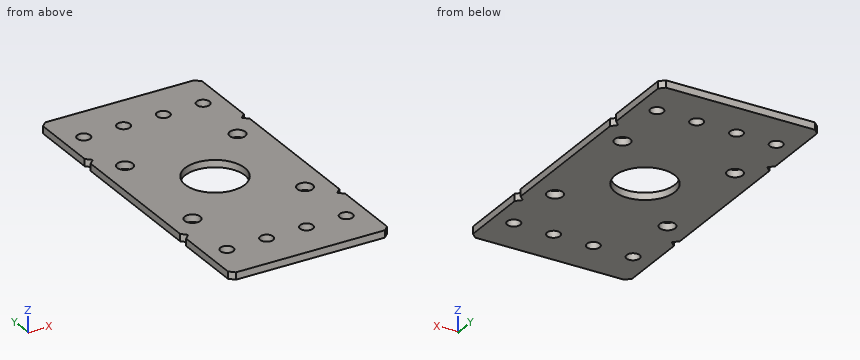
from build123d import *

# Parameters (mm, degrees)
SKETCH1_R           = 2.4892
SKETCH1_R_2         = 2.0701
SKETCH1_R_3         = 9.525
BOSS_EXTRUDE1_DEPTH = 2.286


with BuildPart() as part:
    # Sketch1 → Boss-Extrude1 (new body)
    with BuildSketch(Plane.XY.offset(2.286)):
        Polygon((25.4, -26.9875), (23.8125, -25.4), (25.4, -23.8125), (25.4, 23.8125), (23.8125, 25.4), (25.4, 26.9875), (25.4, 49.2125), (23.8125, 50.8), (-23.8125, 50.8), (-25.4, 49.2125), (-25.4, 26.9875), (-23.8125, 25.4), (-25.4, 23.8125), (-25.4, -23.8125), (-23.8125, -25.4), (-25.4, -26.9875), (-25.4, -49.2125), (-23.8125, -50.8), (23.8125, -50.8), (25.4, -49.2125), align=None)
        with Locations((-17.960512242, -17.960512242)):
            Circle(SKETCH1_R, mode=Mode.SUBTRACT)
        with Locations((-19.05, -38.1)):
            Circle(SKETCH1_R_2, mode=Mode.SUBTRACT)
        with Locations((-6.35, -38.1)):
            Circle(SKETCH1_R_2, mode=Mode.SUBTRACT)
        with Locations((19.05, -38.1)):
            Circle(SKETCH1_R_2, mode=Mode.SUBTRACT)
        Circle(SKETCH1_R_3, mode=Mode.SUBTRACT)
        with Locations((6.35, 38.1)):
            Circle(SKETCH1_R_2, mode=Mode.SUBTRACT)
        with Locations((-19.05, 38.1)):
            Circle(SKETCH1_R_2, mode=Mode.SUBTRACT)
        with Locations((-6.35, 38.1)):
            Circle(SKETCH1_R_2, mode=Mode.SUBTRACT)
        with Locations((19.05, 38.1)):
            Circle(SKETCH1_R_2, mode=Mode.SUBTRACT)
        with Locations((-17.960512242, 17.960512242)):
            Circle(SKETCH1_R, mode=Mode.SUBTRACT)
        with Locations((6.35, -38.1)):
            Circle(SKETCH1_R_2, mode=Mode.SUBTRACT)
        with Locations((17.960512242, -17.960512242)):
            Circle(SKETCH1_R, mode=Mode.SUBTRACT)
        with Locations((17.960512242, 17.960512242)):
            Circle(SKETCH1_R, mode=Mode.SUBTRACT)
    extrude(amount=-BOSS_EXTRUDE1_DEPTH)


solid = part.part
Geometry: final body of the model. Coordinates: model frame, mm. Give positions to 0.01 mm unless a question says otherwise; leave off trailing zeros. Loops run counter-clockwise (first coordinate to the right, second up) from the corner with the lowest first, then second, coordinate; pieces in that order, holes last. Notation, with made-up numbers: M 34,57.25 L 80,57.25 A14 ccw 80,76.25 Z; hole C 64,64.25 d8. An arc over 180 degrees is marked long. Put each result on its own line as item: value. Start each with the question number.
1) Cut plane D-D (z = 0.7). Give the number of separate pieces and of enclosed holes in the cut face, then the cut area to 3 significant figures.
2) Contact query for a flat-ended pin moving along its axis: pin 1 (5.5 mm diameter, centred on x = 19.05, y = -38.1, fed in from +Z). Output: stop coordinate, or through.
3) Ray query, line 1 along X through (y, z) = (-38, 1.8); line 2 along Y through (x, z) = (16.5, 1.4); line 3 along Y through (x, z) = (-16, 1.4). Return the intervals inside material, ascending.
4) Cut plane C-C (x = -19.05). Output: boundary loops of the cut face in (y, z).
5) Cut plane A-A (x = 0). Output: boundary loops of the cut face in (y, z) (3 decimals), then the cut area to 3 significant figures.
6) Cut plane B-B (y = 38.1). Output: boundary loops of the cut face in (x, z).
Verdict:
1. separate pieces: 1
1. enclosed holes: 13
1. area: 4,680 mm2
2. pin 1: z = 2.29
3. line 1: -25.4 to -21.12, -16.98 to -8.42, -4.28 to 4.28, 8.42 to 16.98, 21.12 to 25.4
3. line 2: -50.8 to -19.98, -15.94 to 15.94, 19.98 to 50.8
3. line 3: -50.8 to -19.49, -16.43 to 16.43, 19.49 to 50.8
4. outline: M -50.8,0 L -40.17,0 L -40.17,2.29 L -50.8,2.29 Z; M -36.03,0 L -20.2,0 L -20.2,2.29 L -36.03,2.29 Z; M -15.72,0 L 15.72,0 L 15.72,2.29 L -15.72,2.29 Z; M 20.2,0 L 36.03,0 L 36.03,2.29 L 20.2,2.29 Z; M 40.17,0 L 50.8,0 L 50.8,2.29 L 40.17,2.29 Z
5. outline: M -50.8,0 L -9.525,0 L -9.525,2.286 L -50.8,2.286 Z; M 9.525,0 L 50.8,0 L 50.8,2.286 L 9.525,2.286 Z
5. area: 189 mm2
6. outline: M -25.4,0 L -21.12,0 L -21.12,2.29 L -25.4,2.29 Z; M -16.98,0 L -8.42,0 L -8.42,2.29 L -16.98,2.29 Z; M -4.28,0 L 4.28,0 L 4.28,2.29 L -4.28,2.29 Z; M 8.42,0 L 16.98,0 L 16.98,2.29 L 8.42,2.29 Z; M 21.12,0 L 25.4,0 L 25.4,2.29 L 21.12,2.29 Z
